Answer from the drawing. Dimensions are ordinates in mm from the lowest x, y and z of the part. Round coordinates to 2 decimals unless told otherwise and drop trailing zeros. Loops run counter-clockwise (first coordinate to the right, second up) from the corner with the lowest first, then second, coordinate; pieces in that order, holes last.
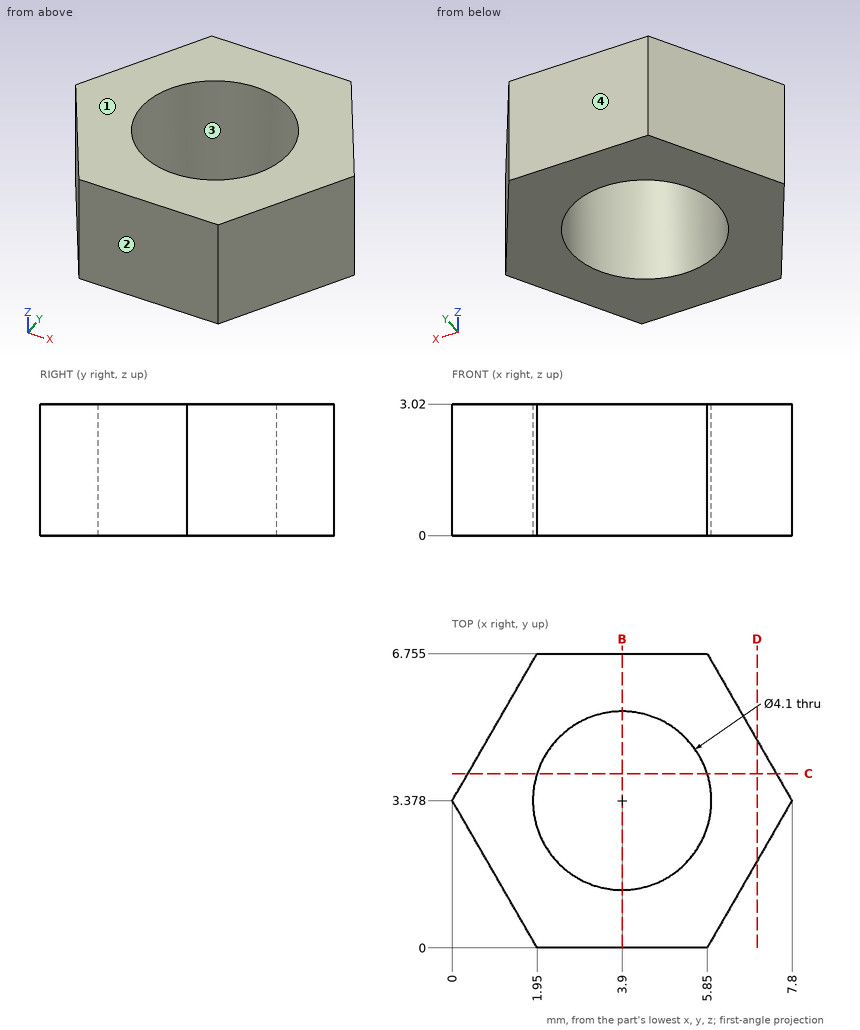
1. Find section D-D (x = 7). Write down the section's boundary in (y, z).
Answer key:
outline: (1.99, 0) - (4.76, 0) - (4.76, 3.02) - (1.99, 3.02) - close
2. Consider probe 1 along Y at (x, z) = (3.9, 1.25) (1 decimal); probe 2 along Y at (x, z) = (3, 1.15) (1 decimal); probe 3 along X at (y, z) = (1.5, 1.2) (1 decimal). Determine where each line is inside the solid, lowest interval first.
Answer key:
probe 1: y = 0 to 1.3, 5.4 to 6.8
probe 2: y = 0 to 1.5, 5.2 to 6.8
probe 3: x = 1.1 to 3.1, 4.7 to 6.7
3. Find section B-B (x = 3.9). Write down the section's boundary in (y, z) (1 decimal).
Answer key:
outline: (0, 0) - (1.3, 0) - (1.3, 3) - (0, 3) - close; (5.4, 0) - (6.8, 0) - (6.8, 3) - (5.4, 3) - close
4. Find section C-C (y = 4). Write down the section's boundary in (x, z).
Answer key:
outline: (0.36, 0) - (1.95, 0) - (1.95, 3.02) - (0.36, 3.02) - close; (5.85, 0) - (7.44, 0) - (7.44, 3.02) - (5.85, 3.02) - close
5. Determine the mould class of the marked faces 1, 2, 3 and 4 for opening direction Y: +Y half, -Y half, draft (parallel to the pull), parting line (faces both ways), or undercut.
Answer key:
face 1: draft
face 2: -Y half
face 3: undercut
face 4: +Y half
